Answer from the drawing. Dimensions are ordinates in mm from the lowest x, y and z of the part. A direction names the side the tool comes from. Give positions to 0.01 mm unless a question says otherwise; leave off trailing zeros. Loops run counter-clockwise (first coordinate to the right, second up) from the corner with the lowest first, then second, coordinate; pieces in that order, holes last. Notation, with made-up numbers: (16, -20.5) -> (64, -20.5) arc R22 ccw to (64, 1.5) -> close; hole circle Ø9 at (7.25, -9.75). An arc over 180 degrees is marked (long way). Answer as CSV lines item,"result". Start each with the question number.
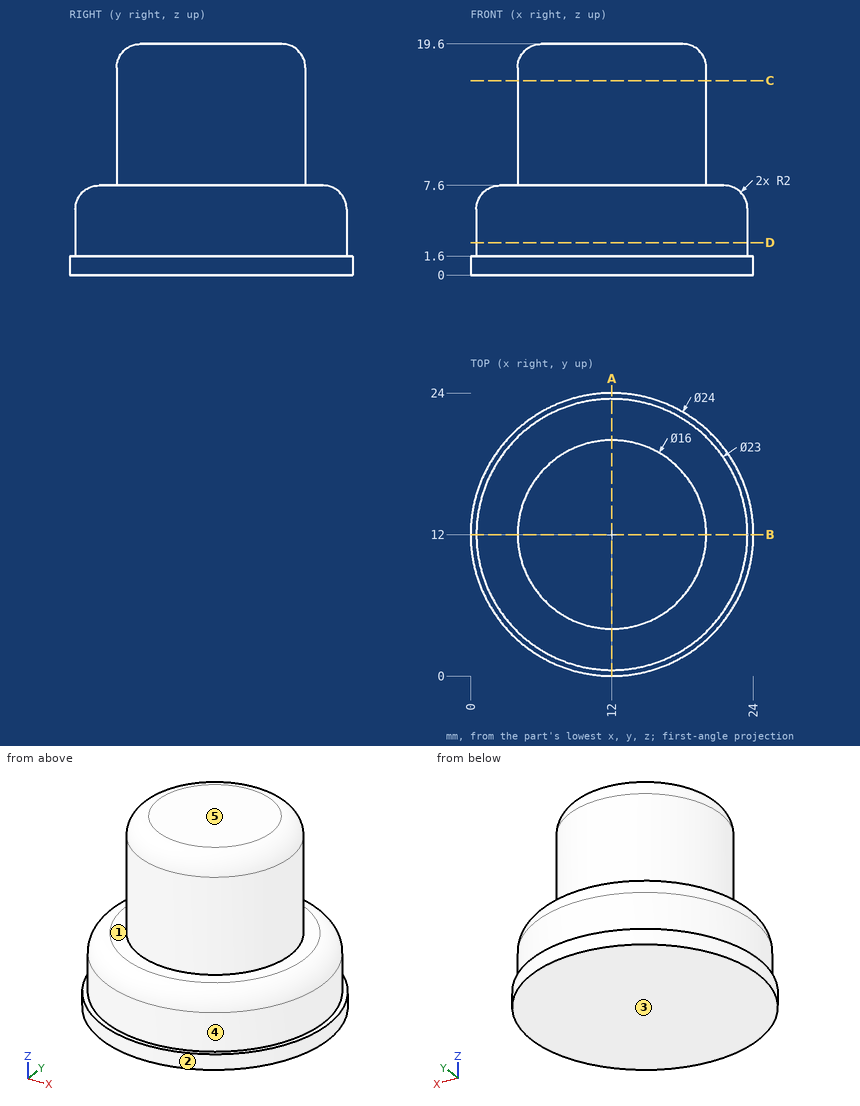
(1) Find section D-D on z = 2.75. Write down the section's boundary in (x, y).
(2) Find the intervals of material crossed by line 1 along Z through (x, y) = (3, 13.5); line 2 along X through (y, z) = (18.25, 11.75); line 3 along Y through (x, z) = (11.75, 17.5), in increasing order. Write a range as from..to.
(3) A tool of negligible diameter and unlimited length cuts with its end or side. For the marked faces 4 and 5, from which of +Z, -Z, +X, -X, +Y, -Y can it reach the whole face along a straight path? Write none if from no direction.
(4) Each of these flat-tipped pins is pushed along its axis until it touches: P1, Ø10, axis at x = 19.5, z = 3, coming from the +Y side; P2, Ø8, axis at x = 21, z = 5.5, coming from the +Y side; P3, Ø8, axis at x = 14.5, z = 5.5, coming from the +Y side. Where does it stop, or does it pass through?
(5) Find section A-A on x = 12. Write down the section's boundary in (y, z).
(6) The mould has two halves that part along Z. Classify the marked faces 1, 2 and 3: pulls with the +Z half, pulls with the -Z half, needs draft (parallel to the pull), parting line crosses it, or undercut.
(7) Find section C-C on z = 16.5. Write down the section's boundary in (x, y), then the cut area to 3 significant figures.
Answer block:
1,outline,"circle Ø23 at (12, 12)"
2,line 1,"z = 0..7.6"
2,line 2,"x = 7.01..16.99"
2,line 3,"y = 4..20"
3,face 4,"+Z"
3,face 5,"+Z, +X, -X, +Y, -Y"
4,P1,"stops at y = 23.69"
4,P2,"stops at y = 22.36"
4,P3,"stops at y = 23.89"
5,outline,"(0, 0) -> (24, 0) -> (24, 1.6) -> (23.5, 1.6) -> (23.5, 5.6) arc R2 ccw to (21.5, 7.6) -> (20, 7.6) -> (20, 17.6) arc R2 ccw to (18, 19.6) -> (6, 19.6) arc R2 ccw to (4, 17.6) -> (4, 7.6) -> (2.5, 7.6) arc R2 ccw to (0.5, 5.6) -> (0.5, 1.6) -> (0, 1.6) -> close"
6,face 1,"pulls with the +Z half"
6,face 2,"needs draft"
6,face 3,"pulls with the -Z half"
7,outline,"circle Ø16 at (12, 12)"
7,area,"201 mm2"
